```python
from build123d import *

# Parameters (mm, degrees)
EXTRUDE_1_DEPTH     = 3
SKETCH_2_R          = 2.025
CUT_EXTRUDE_1_DEPTH = 3
EXTRUDE_2_DEPTH     = 3
FILLET_1_R          = 2


with BuildPart() as part:
    # 草图1 → 凸台-拉伸1 (new body)
    with BuildSketch(Plane.XY):
        Polygon((0, 0), (0, 65), (20, 65), (20, 20), (65, 20), (65, 0), align=None)
    extrude(amount=EXTRUDE_1_DEPTH)

    # 草图2 → 切除-拉伸1 (cut)
    with BuildSketch(Plane.XY.offset(3)):
        with Locations((10, 59)):
            Circle(SKETCH_2_R)
        with Locations((10, 34.5)):
            Circle(SKETCH_2_R)
        with Locations((10, 10)):
            Circle(SKETCH_2_R)
        with Locations((34.5, 10)):
            Circle(SKETCH_2_R)
        with Locations((59, 10)):
            Circle(SKETCH_2_R)
    extrude(amount=-CUT_EXTRUDE_1_DEPTH, mode=Mode.SUBTRACT)

    # 草图3 → 凸台-拉伸2 (add)
    with BuildSketch(Plane.XY.offset(3)):
        Polygon((20, 65), (65, 20), (57.928932188, 20), (20, 57.928932188), align=None)
    extrude(amount=-EXTRUDE_2_DEPTH)

    # 圆角1
    fillet_1_edges = [part.edges().sort_by_distance(p)[0] for p in [
        (0, 0, 1.5),
        (0, 65, 1.5),
        (20, 65, 1.5),
        (20, 20, 1.5),
        (65, 20, 1.5),
        (65, 0, 1.5),
        (57.928932188, 20, 1.5),
        (20, 57.928932188, 1.5),
    ]]
    fillet(fillet_1_edges, radius=FILLET_1_R)


solid = part.part
```
Source: CAD feature listing. Evaluate the final solid. Frame: model axes, mm. A direction names the side the tool comes from. Give positions to 0.01 mm unless a question says otherwise; leave off trailing zeros. Loops run counter-clockwise (first coordinate to the right, second up) from the corner with the lowest first, then second, coordinate; pieces in that order, holes last. Notation, with made-up numbers: (-21.5, -1.5) - (3.5, -1.5) arc R30 cw to (3.5, 28.5) - close; hole circle Ø5 at (36.25, 28). An arc over 180 degrees is marked (long way). Use CSV: the item, a comma, the result in double quotes. Start each with the question number.
1. Reachability of faces 4 (the cylindrical face through (64.844, 19.947, 1.521)), 5 (the flat face through (37, 20, 1)) from +Z, -Z, +X, -X, +Y, -Y: full face, straight path, thin tool, end or side. Return the list, or none.
2. Section A-A (y = 10). Output: boundary loops of the cut face in (x, z) (3 decimals), then the cut area to 3 significant figures.
3. Draft query along X for faces 1 (the cylindrical face through (0.6, 64.43, 1.52)), 2 (the cylindrical face through (60.87, 9.22, 1.52)), 3 (the cylindrical face through (19.947, 64.844, 1.521)). Return one class per face: +X half, -X half, draft (parallel to the pull), parting line (faces both ways), or undercut.
4. Section C-C (z = 1). Count the separate pieces of the cut face and the enclosed holes in it, then the cut area to 3 significant figures.
5. Pin query (flat end, axial travel): pin 1 (8 mm diameter, centred on x = 11.5, y = 56.5, fed in from -Z); pin 2 (0.9 mm diameter, centred on y = 37, z = 1.5, fed in from +X). Return the tip coordinate at first contact, or that it passes through.
6. Section B-B (x = 59). Output: boundary loops of the cut face in (y, z) (3 decimals).
7. Ray query, L1, parallel to Y at x = 10, z = 1.75 (3 decimals); L2, parallel to Y at x = 9, z = 1; L3, parallel to X at y = 33, z = 1.4. Return the intervals inside material, ascending.
Response:
1,face 4,"+Z, -Z, +X, +Y"
1,face 5,"+Z, -Z"
2,outline,"(0, 0) - (7.975, 0) - (7.975, 3) - (0, 3) - close; (12.025, 0) - (32.475, 0) - (32.475, 3) - (12.025, 3) - close; (36.525, 0) - (56.975, 0) - (56.975, 3) - (36.525, 3) - close; (61.025, 0) - (65, 0) - (65, 3) - (61.025, 3) - close"
2,area,"159 mm²"
3,face 1,"-X half"
3,face 2,"undercut"
3,face 3,"+X half"
4,separate pieces,"1"
4,enclosed holes,"6"
4,area,"2,440 mm²"
5,pin 1,"z = 0"
5,pin 2,"x = 48.45"
6,outline,"(0, 0) - (7.975, 0) - (7.975, 3) - (0, 3) - close; (12.025, 0) - (26, 0) - (26, 3) - (12.025, 3) - close"
7,L1,"0 to 7.975, 12.025 to 32.475, 36.525 to 56.975, 61.025 to 65"
7,L2,"0 to 8.24, 11.76 to 32.74, 36.26 to 57.24, 60.76 to 65"
7,L3,"0 to 8.64, 11.36 to 20, 44.93 to 52"
